Build history of the part. All positions in model axes, mm. Give positions to 0.01 mm unless a question says otherwise; leave off trailing zeros. Order: outer loops, then holes, each group sorted by start corner. A loop starts at its lowest first (then second) coordinate and runs counter-clockwise, first axis right, second up. Notation, with made-up numbers: (68, 48) - (111, 48) arc R28 cw to (111, 70) - close; hole circle Ø4 at (65, -35.75). An arc over 180 degrees is marked (long way). Use a Markdown table: item, result. Add a question column.
(1) Slice it at C-C (z = -0.85). Write the cut outline in (x, y) (3 decimals).
(2) Slice it at D-D (y = 5.75). Write the cut outline in (x, z), then the cut area to 3 significant figures.
(3) Slice it at A-A (y = 12.7). Write the cut outline in (x, z), then the cut area to 3 significant figures.
(4) Wall check: line 1 (X direction, y = 13.5, z = -1.4); line 2 (X direction, y = 6, z = -0.1); line 3 (Y direction, x = 12.25, z = -0.85). Give the ranges that are in metal, low to high.
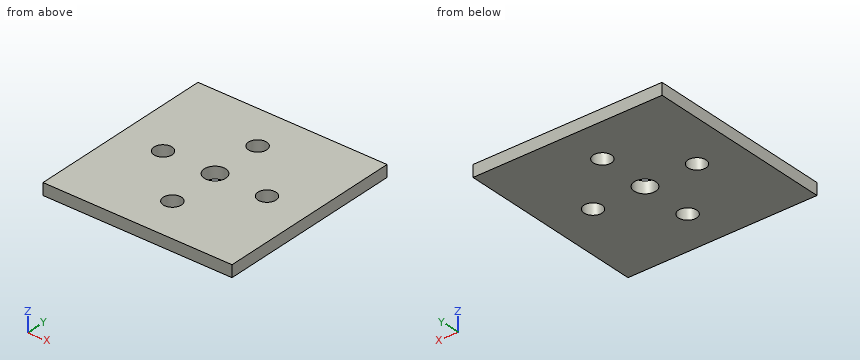
from build123d import *

# Parameters (mm, degrees)
SKETCH1_W              = 25.4
SKETCH1_H              = 25.4
BASE_FLANGE1_DEPTH     = 1.5875
M2_5_CLEARANCE_HOLE1_D = 2.9
F_2_CLEARANCE_HOLE1_D  = 2.4384
CIRPATTERN1_COUNT      = 4


# Sheet-metal steps are written as plain solids
with BuildPart() as part:
    # Sketch1 → Base-Flange1 (new body)
    with BuildSketch(Plane.XY):
        with Locations((12.7, 12.7)):
            Rectangle(SKETCH1_W, SKETCH1_H)
    extrude(amount=-BASE_FLANGE1_DEPTH)

    # M2.5 Clearance Hole1 (through all)
    with Locations(Plane.XY):
        with Locations((12.7, 12.7)):
            Hole(M2_5_CLEARANCE_HOLE1_D / 2)

    # #2 Clearance Hole1 (through all)
    with Locations(Plane.XY):
        with Locations((19.685, 12.7)):
            f_2_clearance_hole1 = Hole(F_2_CLEARANCE_HOLE1_D / 2)

    # CirPattern1: #2 Clearance Hole1 ×4 about axis
    cirpattern1_axis = Axis((12.7, 12.7, 0), (0, 0, 1))
    for i in range(1, CIRPATTERN1_COUNT):
        add(f_2_clearance_hole1.rotate(cirpattern1_axis, i * 360 / CIRPATTERN1_COUNT), mode=Mode.SUBTRACT)


solid = part.part
Solution:
| question | item | result |
|---|---|---|
| 1 | outline | (0, 0) - (25.4, 0) - (25.4, 25.4) - (0, 25.4) - close; hole circle Ø2.438 at (5.715, 12.7); hole circle Ø2.9 at (12.7, 12.7); hole circle Ø2.438 at (12.7, 5.715); hole circle Ø2.438 at (12.7, 19.685); hole circle Ø2.438 at (19.685, 12.7) |
| 2 | outline | (0, -1.59) - (11.48, -1.59) - (11.48, 0) - (0, 0) - close; (13.92, -1.59) - (25.4, -1.59) - (25.4, 0) - (13.92, 0) - close |
| 2 | area | 36.5 mm2 |
| 3 | outline | (0, -1.59) - (4.5, -1.59) - (4.5, 0) - (0, 0) - close; (6.93, -1.59) - (11.25, -1.59) - (11.25, 0) - (6.93, 0) - close; (14.15, -1.59) - (18.47, -1.59) - (18.47, 0) - (14.15, 0) - close; (20.9, -1.59) - (25.4, -1.59) - (25.4, 0) - (20.9, 0) - close |
| 3 | area | 28.0 mm2 |
| 4 | line 1 | 0 to 4.79, 6.64 to 11.49, 13.91 to 18.76, 20.61 to 25.4 |
| 4 | line 2 | 0 to 11.51, 13.89 to 25.4 |
| 4 | line 3 | 0 to 4.58, 6.85 to 11.32, 14.08 to 18.55, 20.82 to 25.4 |
